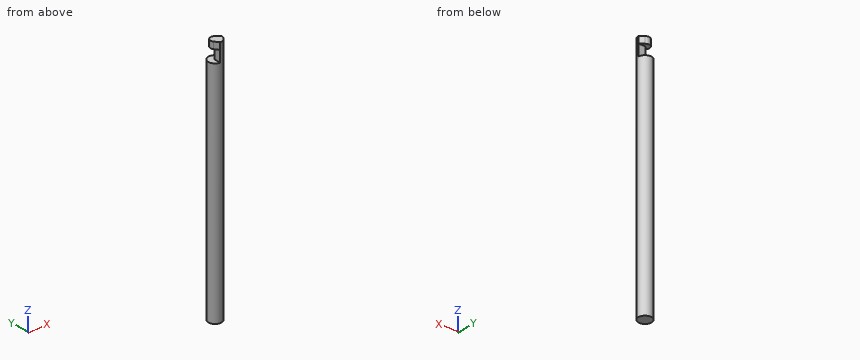
from build123d import *

# Parameters (mm, degrees)
SKETCH1_W          = 55
SKETCH1_H          = 1.5
CUT_EXTRUDE1_START = -4
CUT_EXTRUDE1_DEPTH = 2.5
CUT_EXTRUDE2_START = -1.5
CUT_EXTRUDE2_DEPTH = 1.5


with BuildPart() as part:
    # Sketch1 → Revolve1 (revolve)
    with BuildSketch(Plane(origin=(0, 0, 0), x_dir=(0, 0, -1), z_dir=(1, 0, 0)), mode=Mode.PRIVATE) as revolve1_sk:
        with Locations((27.5, 0.75)):
            Rectangle(SKETCH1_W, SKETCH1_H)
    revolve(revolve1_sk.sketch.rotate(Axis((0, 0, 9.840994653), (0, 0, -1)), 180), axis=Axis((0, 0, 9.840994653), (0, 0, -1)))

    # Sketch2 → Cut-Extrude1 (cut)
    with BuildSketch(Plane.XY.offset(CUT_EXTRUDE1_START)):
        with BuildLine():
            Line((0, 0.1), (1.496662955, 0.1))
            ThreePointArc((1.496662955, 0.1), (-1.060660172, 1.060660172), (-0.1, -1.496662955))
            Line((-0.1, -1.496662955), (-0.1, 0))
            ThreePointArc((-0.1, 0), (-0.070710678, 0.070710678), (0, 0.1))
        make_face()
    extrude(amount=CUT_EXTRUDE1_DEPTH, mode=Mode.SUBTRACT)

    # Sketch3 → Cut-Extrude2 (cut)
    with BuildSketch(Plane.XY.offset(CUT_EXTRUDE2_START)):
        with BuildLine():
            Line((1.496662955, 0.1), (0.615493136, 0.788142246))
            ThreePointArc((0.615493136, 0.788142246), (-0.707106781, 0.707106781), (-0.788142246, -0.615493136))
            Line((-0.788142246, -0.615493136), (-0.1, -1.496662955))
            ThreePointArc((-0.1, -1.496662955), (-1.060660172, 1.060660172), (1.496662955, 0.1))
        make_face()
    extrude(amount=CUT_EXTRUDE2_DEPTH, mode=Mode.SUBTRACT)


solid = part.part
The listing builds one solid part. Answer for the finished solid, in the listing's coordinates (mm). Give positions to 0.01 mm unless a question says otherwise; leave off trailing zeros. Write each loop counter-clockwise with the first axis right and the second up, starting at its lowest first coordinate (ties: lowest second). Pieces come first, ordered by that corner, then holes. Notation, with made-up numbers: (36.5, 12.5) -> (49.5, 12.5) arc R19 ccw to (49.5, 38.5) -> close; hole circle Ø9 at (88, 43). An arc over 180 degrees is marked (long way). Use a Markdown table: item, result.
(1) Find the intervals of material crossed by probe 1 along X at (y, z) = (-0.2, -37.5); probe 2 along Z at (x, y) = (1.1, 0.9); probe 3 along Y at (x, z) = (-0.85, -50.5), in increasing order. Write a range as from..to.
Return value:
| item | result |
|---|---|
| probe 1 | -1.49..1.49 |
| probe 2 | -55..-4 |
| probe 3 | -1.24..1.24 |
(2) Flat-ended cylindrical pins translate along their axes: P1, Ø1.2, axis at y = -1, z = -2.5, coming from the -X side; P2, Ø1.5, axis at x = -1, z = -15, coming from the +Y side. Find the tip coordinate at first contact, or state that the pin passes through.
Return value:
| item | result |
|---|---|
| P1 | x = -0.1 |
| P2 | y = 1.48 |
(3) Section A-A, the plane z = -21 is taken. Determine the outline of the cut face in (x, y), then the cut area to 3 significant figures.
Return value:
| item | result |
|---|---|
| outline | circle Ø3 at (0, 0) |
| area | 7.07 mm2 |
